```python
from build123d import *

# Parameters (mm, degrees)
F1_W     = 60
F1_H     = 60
F2_DEPTH = 2
F0_R     = 0.3
F3_DEPTH = 2
F4_R     = 15
F5_W     = 30
F5_H     = 42.5
F6_DEPTH = 2
F7_R     = 6
F9_DEPTH = 15


with BuildPart() as f2:
    # F1 (on Front) → F2 (new body)
    with BuildSketch(Plane.XZ):
        Rectangle(F1_W, F1_H)
    extrude(amount=-F2_DEPTH)

    # F0 (on Front) → F3 (cut)
    with BuildSketch(Plane.XZ):
        with Locations((-21.7804442346, 18.32)):
            Circle(F0_R)
        with Locations((-21.7804442346, 15.78)):
            Circle(F0_R)
        with Locations((-21.7804442346, 12.62)):
            Circle(F0_R)
        with Locations((-21.7804442346, 10.08)):
            Circle(F0_R)
        with Locations((-21.7804442346, 6.92)):
            Circle(F0_R)
        with Locations((-21.7804442346, 4.38)):
            Circle(F0_R)
        with Locations((-21.7804442346, 1.22)):
            Circle(F0_R)
        with Locations((-21.7804442346, -1.32)):
            Circle(F0_R)
        with Locations((-21.7804442346, -4.48)):
            Circle(F0_R)
        with Locations((-21.7804442346, -7.02)):
            Circle(F0_R)
        with Locations((-21.7804442346, -10.18)):
            Circle(F0_R)
        with Locations((-21.7804442346, -12.72)):
            Circle(F0_R)
        with Locations((-21.7804442346, -15.88)):
            Circle(F0_R)
        with Locations((-21.7804442346, -18.42)):
            Circle(F0_R)
        with Locations((21.6231053323, 18.5572249132)):
            Circle(F0_R)
        with Locations((21.6231053323, 16.0172249132)):
            Circle(F0_R)
        with Locations((21.6231053323, 12.8572249132)):
            Circle(F0_R)
        with Locations((21.6231053323, 10.3172249132)):
            Circle(F0_R)
        with Locations((21.6231053323, 7.1572249132)):
            Circle(F0_R)
        with Locations((21.6231053323, 4.6172249132)):
            Circle(F0_R)
        with Locations((21.6231053323, 1.4572249132)):
            Circle(F0_R)
        with Locations((21.6231053323, -1.0827750868)):
            Circle(F0_R)
        with Locations((21.6231053323, -4.2427750868)):
            Circle(F0_R)
        with Locations((21.6231053323, -6.7827750868)):
            Circle(F0_R)
        with Locations((21.6231053323, -9.9427750868)):
            Circle(F0_R)
        with Locations((21.6231053323, -12.4827750868)):
            Circle(F0_R)
        with Locations((21.6231053323, -15.6427750868)):
            Circle(F0_R)
        with Locations((21.6231053323, -18.1827750868)):
            Circle(F0_R)
        with Locations((-18.5336389446, 20.8555777156)):
            Circle(F0_R)
        with Locations((-15.9936389446, 20.8555777156)):
            Circle(F0_R)
        with Locations((-12.8336389446, 20.8555777156)):
            Circle(F0_R)
        with Locations((-10.2936389446, 20.8555777156)):
            Circle(F0_R)
        with Locations((-7.1336389446, 20.8555777156)):
            Circle(F0_R)
        with Locations((-4.5936389446, 20.8555777156)):
            Circle(F0_R)
        with Locations((-1.4336389446, 20.8555777156)):
            Circle(F0_R)
        with Locations((1.1063610554, 20.8555777156)):
            Circle(F0_R)
        with Locations((4.2663610554, 20.8555777156)):
            Circle(F0_R)
        with Locations((6.8063610554, 20.8555777156)):
            Circle(F0_R)
        with Locations((9.9663610554, 20.8555777156)):
            Circle(F0_R)
        with Locations((12.5063610554, 20.8555777156)):
            Circle(F0_R)
        with Locations((15.6663610554, 20.8555777156)):
            Circle(F0_R)
        with Locations((18.2063610554, 20.8555777156)):
            Circle(F0_R)
    extrude(amount=-F3_DEPTH, mode=Mode.SUBTRACT)

    # F4
    f4_edges = [f2.edges().sort_by_distance(p)[0] for p in [
        (-30, 1, 30),
        (30, 1, 30),
        (30, 1, -30),
        (-30, 1, -30),
    ]]
    fillet(f4_edges, radius=F4_R)

    # F5 (on face) → F6 (cut)
    with BuildSketch(Plane.XZ):
        with Locations((0, -8.75)):
            Rectangle(F5_W, F5_H)
    extrude(amount=-F6_DEPTH, mode=Mode.SUBTRACT)

    # F7
    f7_edges = [f2.edges().sort_by_distance(p)[0] for p in [
        (15, 1, -30),
        (-15, 1, -30),
        (-15, 1, 12.5),
        (15, 1, 12.5),
    ]]
    fillet(f7_edges, radius=F7_R)

    # F8 (on face) → F9 (join)
    with BuildSketch(Plane.XZ):
        with BuildLine():
            ThreePointArc((-24, -25.0623058987), (-27.3237575439, -20.5113519213), (-28.5, -15))
            Line((-28.5, -15), (-28.5, 15))
            ThreePointArc((-28.5, 15), (-24.545941546, 24.545941546), (-15, 28.5))
            Line((-15, 28.5), (15, 28.5))
            ThreePointArc((15, 28.5), (24.545941546, 24.545941546), (28.5, 15))
            Line((28.5, 15), (28.5, -15))
            ThreePointArc((28.5, -15), (27.3237575439, -20.5113519213), (24, -25.0623058987))
            Line((24, -25.0623058987), (25, -26.1803398875))
            ThreePointArc((25, -26.1803398875), (28.6930639376, -21.123724357), (30, -15))
            Line((30, -15), (30, 15))
            ThreePointArc((30, 15), (25.6066017178, 25.6066017178), (15, 30))
            Line((15, 30), (-15, 30))
            ThreePointArc((-15, 30), (-25.6066017178, 25.6066017178), (-30, 15))
            Line((-30, 15), (-30, -15))
            ThreePointArc((-30, -15), (-28.6930639376, -21.123724357), (-25, -26.1803398875))
            Line((-25, -26.1803398875), (-24, -25.0623058987))
        make_face()
    extrude(amount=F9_DEPTH)


solid = f2.part
```
For this review, take the finished solid that the model builds, in its own axes (mm). A direction names the side the tool comes from. Coordinates: 2 decimals unless noted, no trailing zeros. Order: outer loops, then holes, each group sorted by start corner. A loop starts at its lowest first (then second) coordinate and runs counter-clockwise, first axis right, second up. Notation, with made-up numbers: (-31.75, -13) -> (-11.75, -13) arc R5 ccw to (-11.75, -5) -> close; hole circle Ø1 at (-37, 36.25). An arc over 180 degrees is marked (long way). Use CSV: the item, a comma, the result in double quotes. Start each with the question number.
Item 1: Insertion check: pin 1 (2 mm diameter, centred on x = 2.5, y = 1.5, fed in from -Z); pin 2 (5 mm diameter, centred on x = -11, y = -1.5, fed in from -Z); pin 3 (5 mm diameter, centred on x = -13, z = 15, fed in from -Y). Each pin has a flat end and moves straight along its axis. Give the tip position at first contact, or say it passes through.
Item 2: We need section C-C, the plane z = 22.5. Give the boundary of the cut face in (x, y).
Item 3: We need section B-B, the plane x = 11.5. Give the boundary of the cut face in (y, z).
Item 4: Draft analysis for pull direction Z (two halves, no side actions). For faces 4 (the face through (28.5, -7, 0)), 5 (the face through (0, 2, 14)), 6 (the face through (0, -7, 28.5)), state which applies: pulls with the +Z half, pulls with the -Z half, needs draft (parallel to the pull), parting line crosses it, or undercut.
Item 5: We need section A-A, the plane y = -11.75. Give the boundary of the cut face in (x, z), then the cut area to 3 significant figures.
Item 6: For faces 1 (the face through (0, -6, 30)), 2 (the face through (0, 1, 12.5)), 3 (the face through (-28.5, -7, 0)), list the 3-axis set-ups (+Z, -Z, +X, -X, +Y, -Y) from which the entire face can be reached by the end or side of a thin tool; tool diameter is ignored.
Item 7: Wall thickness on probe 1 along X at (y, z) = (-1.5, 5.5); probe 2 along Z at (x, y) = (1, -5.25); probe 3 along Y at (x, z) = (24.5, -19.5): over which ranges is each line inside the solid? List them lowest first.
Derived:
1,pin 1,"stops at z = 12.5"
1,pin 2,"stops at z = 10.97"
1,pin 3,"stops at y = 0"
2,outline,"(-27.99, -15) -> (-26.22, -15) -> (-26.22, 0) -> (26.22, 0) -> (26.22, -15) -> (27.99, -15) -> (27.99, 2) -> (-27.99, 2) -> close"
3,outline,"(-15, 28.5) -> (0, 28.5) -> (0, 11.95) -> (2, 11.95) -> (2, 30) -> (-15, 30) -> close"
4,face 4,"undercut"
4,face 5,"needs draft"
4,face 6,"pulls with the -Z half"
5,outline,"(-30, -15) arc R15 ccw to (-25, -26.18) -> (-24, -25.06) arc R13.5 cw to (-28.5, -15) -> (-28.5, 15) arc R13.5 cw to (-15, 28.5) -> (15, 28.5) arc R13.5 cw to (28.5, 15) -> (28.5, -15) arc R13.5 cw to (24, -25.06) -> (25, -26.18) arc R15 ccw to (30, -15) -> (30, 15) arc R15 ccw to (15, 30) -> (-15, 30) arc R15 ccw to (-30, 15) -> close"
5,area,"238 mm^2"
6,face 1,"+Z, +X, -X, +Y, -Y"
6,face 2,"-Z, +Y, -Y"
6,face 3,"-Y"
7,probe 1,"x = -30 to -28.5, 28.5 to 30"
7,probe 2,"z = 28.5 to 30"
7,probe 3,"y = 0 to 2"
